```python
from build123d import *

# Parameters (mm, degrees)
F0_W     = 40
F0_H     = 40
F1_DEPTH = 40
F2_W     = 15
F2_H     = 15
F3_DEPTH = 40.001
F4_W     = 15
F4_H     = 15
F5_DEPTH = 40.001
F6_W     = 15
F6_H     = 15
F7_DEPTH = 40.001


with BuildPart() as f1:
    # F0 (on Front) → F1 (new body)
    with BuildSketch(Plane.XZ):
        Rectangle(F0_W, F0_H)
    extrude(amount=F1_DEPTH)

    # F2 (on face) → F3 (cut, through all)
    with BuildSketch(Plane.XZ.offset(40)):
        with Locations((-10, 10)):
            Rectangle(F2_W, F2_H)
        with Locations((10, 10)):
            Rectangle(F2_W, F2_H)
        with Locations((-10, -10)):
            Rectangle(F2_W, F2_H)
        with Locations((10, -10)):
            Rectangle(F2_W, F2_H)
    extrude(amount=-F3_DEPTH, mode=Mode.SUBTRACT)

    # F4 (on face) → F5 (cut, through all)
    with BuildSketch(Plane(origin=(-20, 0, 0), x_dir=(0, -1, 0), z_dir=(-1, 0, 0))):
        with Locations((10, 10)):
            Rectangle(F4_W, F4_H)
        with Locations((30, 10)):
            Rectangle(F4_W, F4_H)
        with Locations((10, -10)):
            Rectangle(F4_W, F4_H)
        with Locations((30, -10)):
            Rectangle(F4_W, F4_H)
    extrude(amount=-F5_DEPTH, mode=Mode.SUBTRACT)

    # F6 (on face) → F7 (cut, through all)
    with BuildSketch(Plane.XY.offset(20)):
        with Locations((-10, -10)):
            Rectangle(F6_W, F6_H)
        with Locations((10, -10)):
            Rectangle(F6_W, F6_H)
        with Locations((-10, -30)):
            Rectangle(F6_W, F6_H)
        with Locations((10, -30)):
            Rectangle(F6_W, F6_H)
    extrude(amount=-F7_DEPTH, mode=Mode.SUBTRACT)


solid = f1.part
```
The model under review builds one solid part; all positions refer to its coordinate system, in mm. A direction names the side the tool comes from. Round coordinates to 2 decimals unless told otherwise and drop trailing zeros. Loops run counter-clockwise (first coordinate to the right, second up) from the corner with the lowest first, then second, coordinate; pieces in that order, holes last. Notation, with made-up numbers: M -19.75,-5.5 L -3.75,-5.5 A32 ccw -3.75,31.5 Z; hole C 6,28 d1. An arc over 180 degrees is marked long. Put each result on its own line as item: value.
Q1. Consider section A-A, the plane z = -1. Give the boundary of the cut face in (x, y), then the cut area to 3 significant figures.
Result set:
outline: M -20,-40 L 20,-40 L 20,0 L -20,0 Z; hole M -17.5,-37.5 L -2.5,-37.5 L -2.5,-22.5 L -17.5,-22.5 Z; hole M -17.5,-17.5 L -2.5,-17.5 L -2.5,-2.5 L -17.5,-2.5 Z; hole M 2.5,-37.5 L 17.5,-37.5 L 17.5,-22.5 L 2.5,-22.5 Z; hole M 2.5,-17.5 L 17.5,-17.5 L 17.5,-2.5 L 2.5,-2.5 Z
area: 700 mm²
Q2. Mouldability with a two-part tool opening along Z and no side actions: class faces 4 (the flat face through (-17.5, -30, 19)), 5 (the flat face through (-5, -20, -20)), 6 (the flat face through (10, -1, -17.5)) as released by +Z, released by -Z, zero draft, split by the parting line, or undercut.
Result set:
face 4: zero draft
face 5: released by -Z
face 6: undercut
Q3. For pin 1 (1 mm diameter, centred on x = 15.5, y = -16.5, fed in from +Z), flat-tipped, find the tip position at first contact; note if it passes through.
Result set:
pin 1: passes through
Q4. To check wall thickness, follow L1, parallel to X at y = -38, z = 7; L2, parallel to Y at x = 1, z = 6.5. State the ranges of each line that lie inside material, in increasing order.
Result set:
L1: x = -20 to -17.5, -2.5 to 2.5, 17.5 to 20
L2: y = -40 to -37.5, -22.5 to -17.5, -2.5 to 0
Q5. Machinability: for faces 1 (the flat face through (-10, -37.5, 0)), 2 (the flat face through (-2.5, -39, -10)), 3 (the flat face through (0, -10, 2.5)), which of the approach directions +Z, -Z, +X, -X, +Y, -Y give a long, thin tool a straight path to every point of the face, cutting with its end or side? Answer none if there is none.
Result set:
face 1: +Z, -Z
face 2: +Y, -Y
face 3: +X, -X
Q6. Consider section C-C, the plane x = -9.5. Count the separate pieces of the cut face and the enclosed holes in it, then the cut area to 3 significant figures.
Result set:
separate pieces: 9
enclosed holes: 0
area: 100 mm²
Q7. Consider section B-B, the plane y = -20.5. Give the boundary of the cut face in (x, z).
Result set:
outline: M -20,-20 L 20,-20 L 20,20 L -20,20 Z; hole M -17.5,-17.5 L -2.5,-17.5 L -2.5,-2.5 L -17.5,-2.5 Z; hole M -17.5,2.5 L -2.5,2.5 L -2.5,17.5 L -17.5,17.5 Z; hole M 2.5,-17.5 L 17.5,-17.5 L 17.5,-2.5 L 2.5,-2.5 Z; hole M 2.5,2.5 L 17.5,2.5 L 17.5,17.5 L 2.5,17.5 Z
